For this review, take the finished solid that the model builds, in its own axes (mm). A direction names the side the tool comes from. Round coordinates to 2 decimals unless told otherwise and drop trailing zeros. Order: outer loops, then holes, each group sorted by start corner. A loop starts at its lowest first (then second) coordinate and runs counter-clockwise, first axis right, second up. Notation, with made-up numbers: M -4,4 L 32,4 A4 ccw 32,9 Z; hole C 0.25,59.5 d5. An arc over 180 degrees is marked long. Use a Markdown table: item, result.
from build123d import *

# Parameters (mm, degrees)
BOSS_EXTRUDE1_DEPTH = 20.32


# Read off the part's stored shape, not the designer's step: #2 Clearance Hole1
with BuildPart() as part:
    # Sketch1 → Boss-Extrude1 (new body)
    with BuildSketch(Plane(origin=(0, 0, 0), x_dir=(1, 0, 0), z_dir=(0, 1, 0))):
        with BuildLine():
            Line((0, 13.208), (0, 9.398))
            ThreePointArc((0, 9.398), (9.398, 0), (0, -9.398))
            Line((0, -9.398), (0, -13.208))
            ThreePointArc((0, -13.208), (13.208, 0), (0, 13.208))
        make_face()
    extrude(amount=BOSS_EXTRUDE1_DEPTH)

    # #2 Clearance Hole1 outline → #2 Clearance Hole1 (revolve, cut)
    with BuildSketch(Plane(origin=(0, 5.08, -11.303), x_dir=(0, 1, 0), z_dir=(0, 0, -1))):
        Polygon((2.0701, 6.833260935), (2.0701, 9.445172288), (0, 9.445172288), (0, 0), (1.1303, 0), (1.1303, 6.044675101), align=None)
    revolve(axis=Axis((0, 5.08, -11.303), (1, 0, 0)), mode=Mode.SUBTRACT)

    # 2 Clearance Hole1 2 outline → 2 Clearance Hole1 2 (revolve, cut)
    with BuildSketch(Plane(origin=(0, 5.08, 11.303), x_dir=(0, 1, 0), z_dir=(0, 0, -1))):
        Polygon((2.0701, 9.445172288), (0, 9.445172288), (0, 0), (1.1303, 0), (1.1303, 6.044675101), (2.0701, 6.833260935), align=None)
    revolve(axis=Axis((0, 5.08, 11.303), (1, 0, 0)), mode=Mode.SUBTRACT)

    # 2 Clearance Hole1 3 outline → 2 Clearance Hole1 3 (revolve, cut)
    with BuildSketch(Plane(origin=(0, 15.24, 11.303), x_dir=(0, 1, 0), z_dir=(0, 0, -1))):
        Polygon((2.0701, 9.445172288), (0, 9.445172288), (0, 0), (1.1303, 0), (1.1303, 6.044675101), (2.0701, 6.833260935), align=None)
    revolve(axis=Axis((0, 15.24, 11.303), (1, 0, 0)), mode=Mode.SUBTRACT)

    # 2 Clearance Hole1 4 outline → 2 Clearance Hole1 4 (revolve, cut)
    with BuildSketch(Plane(origin=(0, 15.24, -11.303), x_dir=(0, 1, 0), z_dir=(0, 0, -1))):
        Polygon((2.0701, 9.445172288), (0, 9.445172288), (0, 0), (1.1303, 0), (1.1303, 6.044675101), (2.0701, 6.833260935), align=None)
    revolve(axis=Axis((0, 15.24, -11.303), (1, 0, 0)), mode=Mode.SUBTRACT)


solid = part.part
Q1. Add section C-C (x = 8.75). Write out the cut boundary in (y, z), then the cut area to 3 significant figures.
Determined:
| item | result |
|---|---|
| outline | M 0,-9.89 L 3.56,-9.89 A2.07 cw 6.6,-9.89 L 13.72,-9.89 A2.07 cw 16.76,-9.89 L 20.32,-9.89 L 20.32,-3.43 L 0,-3.43 Z; M 0,3.43 L 20.32,3.43 L 20.32,9.89 L 16.76,9.89 A2.07 cw 13.72,9.89 L 6.6,9.89 A2.07 cw 3.56,9.89 L 0,9.89 Z |
| area | 257 mm^2 |
Q2. Wall thickness on line 1 along Y through (x, z) = (8.5, 9.75); line 2 along Z through (x, y) = (1.75, 15.24); line 3 along Z through (x, y) = (2.25, 5.08): over which ranges is each line inside the solid? List them lowest first. Write a range as [from, to].
Determined:
| item | result |
|---|---|
| line 1 | y = [0, 3.71], [6.45, 13.87], [16.61, 20.32] |
| line 2 | z = [-13.09, -12.43], [-10.17, -9.23], [9.23, 10.17], [12.43, 13.09] |
| line 3 | z = [-13.01, -12.43], [-10.17, -9.12], [9.12, 10.17], [12.43, 13.01] |
Q3. Clearance check with flat-ended pins moving along their axes: pin 1 (2.5 mm diameter, centred on y = 5.08, z = -11.303, fed in from -X); pin 2 (1.5 mm diameter, centred on x = 7, y = 3.5, fed in from +Z); pin 3 (1.5 mm diameter, centred on x = 8, y = 14.5, fed in from +Z); pin 4 (2.5 mm diameter, centred on y = 15.24, z = 11.303, fed in from +X). State where each tip first meets the part, or that it passes through.
Determined:
| item | result |
|---|---|
| pin 1 | stops at x = 0 |
| pin 2 | stops at z = 11.64 |
| pin 3 | stops at z = 9.87 |
| pin 4 | stops at x = 6.15 |
Q4. Machinability: for faces 1 (the flat face through (0, 10, -11)), 2 (the cylindrical face through (7.867, 5.034, 9.233)), 3 (the cylindrical face through (7.867, 15.286, -9.233)), which of the approach directions +Z, -Z, +X, -X, +Y, -Y give a long, thin tool a straight path to every point of the face, cutting with its end or side? Answer none if there is none.
Determined:
| item | result |
|---|---|
| face 1 | +Z, -Z, -X, +Y, -Y |
| face 2 | +Z, +X |
| face 3 | -Z, +X |
Q5. Add section D-D (z = 11). Give the number of separate pieces and of enclosed holes in the cut face, then the cut area to 3 significant figures.
Determined:
| item | result |
|---|---|
| separate pieces | 3 |
| enclosed holes | 0 |
| area | 113 mm^2 |
Q6. Draft analysis for pull direction Z (two halves, no side actions). For faces 4 (the cylindrical face through (7.867, 5.126, -9.233)), 5 (the cylindrical face through (7.867, 15.194, 9.233)), 6 (the cylindrical face through (3.065, 15.093, -10.182)), 7 (the flat face through (0, 10, 11)), state which applies: pulls with the +Z half, pulls with the -Z half, needs draft (parallel to the pull), parting line crosses it, or undercut.
Determined:
| item | result |
|---|---|
| face 4 | pulls with the -Z half |
| face 5 | pulls with the +Z half |
| face 6 | undercut |
| face 7 | needs draft |
Q7. Add section A-A (x = 1.25). Write out the cut boundary in (y, z), then the cut area to 3 significant figures.
Determined:
| item | result |
|---|---|
| outline | M 0,-13.15 L 20.32,-13.15 L 20.32,-9.31 L 0,-9.31 Z; M 0,9.31 L 20.32,9.31 L 20.32,13.15 L 0,13.15 Z; hole C 5.08,-11.3 d2.26; hole C 5.08,11.3 d2.26; hole C 15.24,-11.3 d2.26; hole C 15.24,11.3 d2.26 |
| area | 140 mm^2 |
Q8. Add section B-B (y = 5.08). Write out the cut boundary in (x, z).
Determined:
| item | result |
|---|---|
| outline | M 0,-13.21 A13.21 ccw 4.46,-12.43 L 0,-12.43 Z; M 0,-10.17 L 6.04,-10.17 L 6.83,-9.23 L 9.44,-9.23 A13.21 ccw 9.44,9.23 L 6.83,9.23 L 6.04,10.17 L 0,10.17 L 0,9.4 A9.4 cw 0,-9.4 Z; M 0,12.43 L 4.46,12.43 A13.21 ccw 0,13.21 Z |
